The listing builds one solid part. Answer for the finished solid, in the listing's coordinates (mm). Coordinates: 2 decimals unless noted, no trailing zeros. Order: outer loops, then holes, each group sorted by start corner. A loop starts at its lowest first (then second) coordinate and runs counter-clockwise, first axis right, second up. Notation, with made-up numbers: (29.5, 6) -> (67.5, 6) arc R33 cw to (67.5, 38) -> close; hole circle Ø1 at (16.5, 88). An arc over 180 degrees is marked (long way). Return JSON: item names as keys, results as strings.
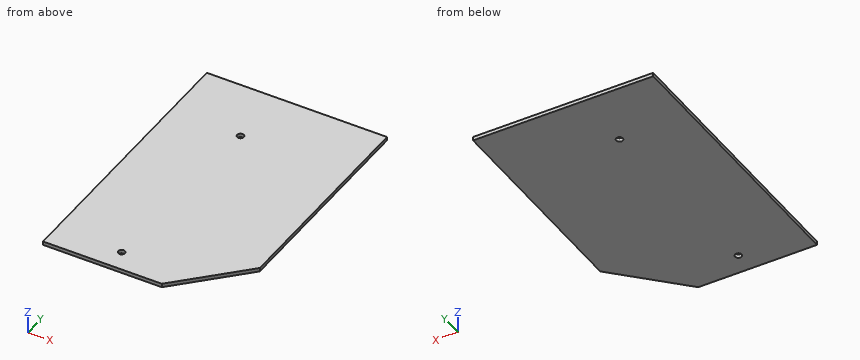
```python
from build123d import *

# Parameters (mm, degrees)
F0_W     = 80.4
F0_H     = 124.25
F1_DEPTH = 1.651
F3_DEPTH = 1.652
F5_D     = 2.9464


with BuildPart() as f1:
    # F0 (on Top) → F1 (new body)
    with BuildSketch(Plane.XY):
        with Locations((40.2, 62.125)):
            Rectangle(F0_W, F0_H)
    extrude(amount=F1_DEPTH)

    # F2 (on face) → F3 (cut, through all)
    with BuildSketch(Plane.XY.offset(1.651)):
        Polygon((80.4, 0), (80.4, 27.75), (53, 0), align=None)
    extrude(amount=-F3_DEPTH, mode=Mode.SUBTRACT)

    # F5 (through all)
    with Locations(Plane.XY.offset(1.651)):
        with Locations((31.5, 96.25), (29.5, 9.5)):
            Hole(F5_D / 2)


solid = f1.part
```
Item 1: The part is cut by section B-B on z = 1.15. Determine the outline of the cut face in (x, y), plus the area to 3 significant figures.
Answer list:
{"outline": "(0, 0) -> (53, 0) -> (80.4, 27.75) -> (80.4, 124.25) -> (0, 124.25) -> close; hole circle Ø2.95 at (29.5, 9.5); hole circle Ø2.95 at (31.5, 96.25)", "area": "9,600 mm2"}
Item 2: The part is cut by section C-C on y = 9.5. Determine the outline of the cut face in (x, z).
Answer list:
{"outline": "(0, 0) -> (28.03, 0) -> (28.03, 1.65) -> (0, 1.65) -> close; (30.97, 0) -> (62.38, 0) -> (62.38, 1.65) -> (30.97, 1.65) -> close"}
Item 3: The part is cut by section A-A on y = 96.25. Determine the outline of the cut face in (x, z).
Answer list:
{"outline": "(0, 0) -> (30.03, 0) -> (30.03, 1.65) -> (0, 1.65) -> close; (32.97, 0) -> (80.4, 0) -> (80.4, 1.65) -> (32.97, 1.65) -> close"}
Item 4: The part is cut by section D-D on x = 74. Determine the outline of the cut face in (y, z).
Answer list:
{"outline": "(21.27, 0) -> (124.25, 0) -> (124.25, 1.65) -> (21.27, 1.65) -> close"}
Item 5: Find the intervals of material crossed by probe 1 along X at (y, z) = (96.25, 1.1); probe 2 along Y at (x, z) = (31.5, 1.05); probe 3 along Y at (x, z) = (29.5, 0.55), in increasing order.
Answer list:
{"probe 1": "0 to 30.03, 32.97 to 80.4", "probe 2": "0 to 94.78, 97.72 to 124.25", "probe 3": "0 to 8.03, 10.97 to 124.25"}
